```python
from build123d import *

# Parameters (mm, degrees)
SZKIC1_W                    = 50
SZKIC1_H                    = 30
DODANIE_WYCI_GNI_CIE1_DEPTH = 5
ZAOKR_GLENIE1_R             = 10
SZKIC2_W                    = 25
SZKIC2_H                    = 20
DODANIE_WYCI_GNI_CIE2_DEPTH = 15
SZKIC3_R                    = 4
WYTNIJ_WYCI_GNI_CIE1_DEPTH  = 30
ZAOKR_GLENIE2_R             = 10


with BuildPart() as part:
    # Szkic1 → Dodanie-wyciągnięcie1 (new body)
    with BuildSketch(Plane(origin=(0, 0, 0), x_dir=(1, 0, 0), z_dir=(0, 1, 0))):
        Rectangle(SZKIC1_W, SZKIC1_H)
    extrude(amount=DODANIE_WYCI_GNI_CIE1_DEPTH)

    # Zaokrąglenie1
    zaokr_glenie1_edges = [part.edges().sort_by_distance(p)[0] for p in [
        (25, 2.5, 15),
        (-25, 2.5, 15),
        (-25, 2.5, -15),
        (25, 2.5, -15),
    ]]
    fillet(zaokr_glenie1_edges, radius=ZAOKR_GLENIE1_R)

    # Szkic2 → Dodanie-wyciągnięcie2 (add)
    with BuildSketch(Plane(origin=(0, 5, 0), x_dir=(1, 0, 0), z_dir=(0, 1, 0))):
        Rectangle(SZKIC2_W, SZKIC2_H)
    extrude(amount=DODANIE_WYCI_GNI_CIE2_DEPTH)

    # Szkic3 → Wytnij-wyciągnięcie1 (cut)
    with BuildSketch(Plane.ZY.offset(12.5)):
        with Locations((0, 12.5)):
            Circle(SZKIC3_R)
    extrude(amount=-WYTNIJ_WYCI_GNI_CIE1_DEPTH, mode=Mode.SUBTRACT)

    # Zaokrąglenie2
    zaokr_glenie2_edges = [part.edges().sort_by_distance(p)[0] for p in [
        (0, 20, 10),
        (0, 20, -10),
    ]]
    fillet(zaokr_glenie2_edges, radius=ZAOKR_GLENIE2_R - 0.0001)  # a hair under: the kernel refuses the full size


solid = part.part
```
Check sheet for the modelled part. Datum: model origin and axes. Units: mm. A direction names the side the tool comes from. Round coordinates to 2 decimals unless told otherwise and drop trailing zeros. Order: outer loops, then holes, each group sorted by start corner. A loop starts at its lowest first (then second) coordinate and runs counter-clockwise, first axis right, second up. Notation, with made-up numbers: (39, -33.5) -> (92, -33.5) arc R23 cw to (92, -8.5) -> close; hole circle Ø7 at (18.5, 74). An arc over 180 degrees is marked (long way). Use CSV: the item, a comma, the result in double quotes.
(1) Cross-section at D-D (y = 4.5). Record the boundary of the cut face in (x, z).
Worked out:
outline,"(-25, -5) arc R10 ccw to (-15, -15) -> (15, -15) arc R10 ccw to (25, -5) -> (25, 5) arc R10 ccw to (15, 15) -> (-15, 15) arc R10 ccw to (-25, 5) -> close"
(2) Depth check by flat-ended pin: pin 1 (12 mm diameter, centred on y = 17, z = 10.5, fed in from +X); pin 2 (9 mm diameter, centred on y = 12.5, z = 0, fed in from -X); pin 3 (2 mm diameter, centred on y = 4, z = -11, fed in from -X). Enter the tip coordinate at first touch or a pass-through.
Worked out:
pin 1,"x = 12.5"
pin 2,"x = -12.5"
pin 3,"x = -23.66"
(3) Cross-section at A-A (z = -3). Record the boundary of the cut face in (x, y).
Worked out:
outline,"(-25, 0) -> (25, 0) -> (25, 5) -> (12.5, 5) -> (12.5, 9.85) -> (-12.5, 9.85) -> (-12.5, 5) -> (-25, 5) -> close; (-12.5, 15.15) -> (12.5, 15.15) -> (12.5, 19.54) -> (-12.5, 19.54) -> close"
(4) Cross-section at B-B (y = 9.25). Record the boundary of the cut face in (x, z), and give its area (3 significant figures).
Worked out:
outline,"(-12.5, -10) -> (12.5, -10) -> (12.5, -2.33) -> (-12.5, -2.33) -> close; (-12.5, 2.33) -> (12.5, 2.33) -> (12.5, 10) -> (-12.5, 10) -> close"
area,"383 mm²"
(5) Tool access check on faces 1 (the face through (-12.5, 9.1, 2.4)), 2 (the face through (0, 7, -10)), 3 (the face through (12.5, 9.1, 2.4)), 4 (the face through (0, 7, 10)), 5 (the face through (-0.175, 16.466, -0.521)). Record the directions out of +Z, -Z, +X, -X, +Y, -Y that give a thin tool (end or side, any length) a straight path to the whole face; none if there is none.
Worked out:
face 1,"+Z, -Z, -X, +Y"
face 2,"-Z, +X, -X, +Y"
face 3,"+Z, -Z, +X, +Y"
face 4,"+Z, +X, -X, +Y"
face 5,"+X, -X"
(6) Material ranges on line 1 along Y through (x, z) = (-1, 0); line 2 along Y through (x, z) = (-20.5, 3.5); line 3 along X through (y, z) = (6.5, -2), recorded low to high. Write a range as from..to.
Worked out:
line 1,"0..8.5, 16.5..20"
line 2,"0..5"
line 3,"-12.5..12.5"
